Study the drawing (mm; zero at the part's minimum x, y, z) and answer. Give positions to 0.01 mm unless a question says otherwise; leave off trailing zeros. Write each loop counter-clockwise with the first axis right and the second up, starting at its lowest first coordinate (ties: lowest second). Pieces come first, ordered by that corner, then holes.
1) Straight lines are drawn through the part: probe 1 along Z at (x, y) = (3.85, 25); probe 2 along Z at (x, y) = (1.35, 25); probe 3 along Y at (x, z) = (3.85, 24.5) (3 decimals). For each, find the intervals that lie inside material, in ascending order.
2) Determine the mould class of the marked faces 1, 2 and 3 for opening direction Z: pulls with the +Z half, pulls with the -Z half, needs draft (parallel to the pull), parting line crosses it, or undercut.
3) Find section C-C (x = 0.75). Determine the outline of the cut face in (y, z), plus the area to 3 significant figures.
4) Find section A-A (z = 25). Determine the outline of the cut face in (x, y), plus the area to 3 significant figures.
5) Given pin 1 Ø4 at (y, z) = (25, 12) entering from -X; pin 2 Ø1.5 at (x, z) = (2.5, 43.5) entering from +Y; pin 3 Ø1 at (x, y) = (2.5, 34.5) entering from -Z, each flat-ended and moving along its own axis, determine where each tip first touches the part or whether it passes through.
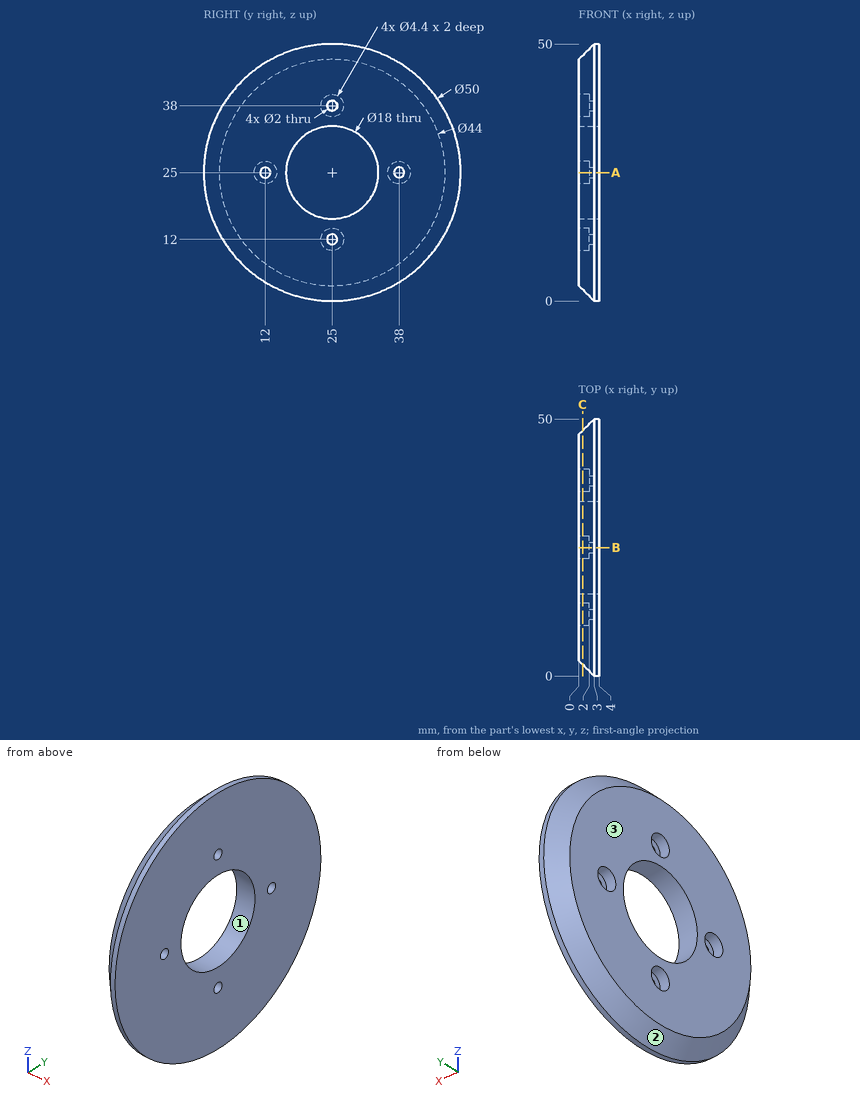
Results:
1. probe 1: z = 0 to 11, 13 to 16, 34 to 37, 39 to 50
1. probe 2: z = 1.65 to 9.8, 14.2 to 16, 34 to 35.8, 40.2 to 48.35
1. probe 3: y = 0.005 to 11.134, 12.866 to 16.014, 33.986 to 37.134, 38.866 to 49.995
2. face 1: undercut
2. face 2: parting line crosses it
2. face 3: needs draft
3. outline: circle Ø45.5 at (25, 25); hole circle Ø4.4 at (12, 25); hole circle Ø18 at (25, 25); hole circle Ø4.4 at (25, 12); hole circle Ø4.4 at (25, 38); hole circle Ø4.4 at (38, 25)
3. area: 1,310 mm2
4. outline: (0, 3) - (3, 0) - (4, 0) - (4, 11) - (2, 11) - (2, 9.8) - (0, 9.8) - close; (0, 14.2) - (2, 14.2) - (2, 13) - (4, 13) - (4, 16) - (0, 16) - close; (0, 34) - (4, 34) - (4, 37) - (2, 37) - (2, 35.8) - (0, 35.8) - close; (0, 40.2) - (2, 40.2) - (2, 39) - (4, 39) - (4, 50) - (3, 50) - (0, 47) - close
4. area: 93.4 mm2
5. pin 1: stops at x = 2
5. pin 2: stops at y = 42.41
5. pin 3: stops at z = 1.84
